Here's the drawing with two shaded views (mm, measured from the low corner). I have some questions. Round coordinates to 2 decimals unless told otherwise and drop trailing zeros. Loops run counter-clockwise (first coordinate to the right, second up) from the corner with the lowest first, then second, coordinate; pieces in that order, holes last. Notation, with made-up numbers: (63.25, 86) -> (75.25, 86) arc R22 ccw to (75.25, 105) -> close; hole circle Ø3 at (6, 56.5). An arc over 180 degrees is marked (long way). Write item = value, one per line.
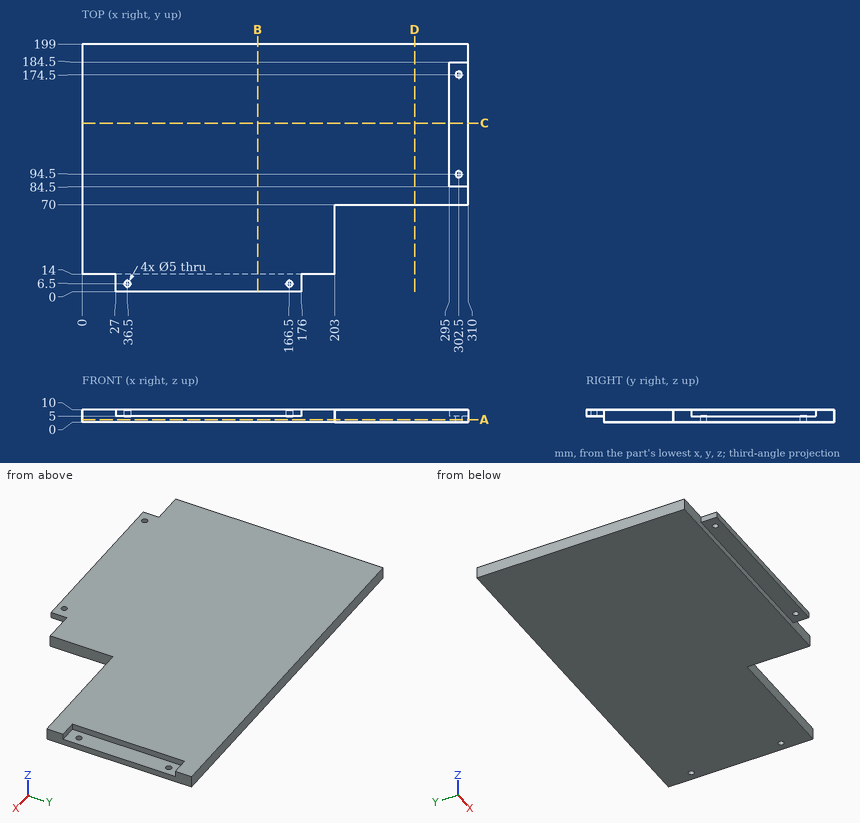
1. Suppose I cut it at A-A, the plane z = 2.25. List the corners of the cut face in (x, y) for me.
Entries:
outline = (0, 14) -> (203, 14) -> (203, 70) -> (310, 70) -> (310, 199) -> (0, 199) -> close; hole circle Ø5 at (302.5, 94.5); hole circle Ø5 at (302.5, 174.5)
2. I need wall thicknesses on line 1 (Y direction, x = 302.5, z = 1.9); line 2 (Y direction, x = 36.5, z = 8.7); line 3 (X direction, y = 144, z = 9.25). Which ranges of each line are inside material? Lowest first, please. Write a range as [from, to].
Entries:
line_1 = [70, 92], [97, 172], [177, 199]
line_2 = [0, 4], [9, 199]
line_3 = [0, 295]
3. Suppose I cut it at C-C, the plane y = 135.5. List the corners of the cut face in (x, z) for me, and give its area (4 significant figures).
Entries:
outline = (0, 0) -> (310, 0) -> (310, 5) -> (295, 5) -> (295, 10) -> (0, 10) -> close
area = 3,025 mm²
4. I'm going to push flat-ended pins straight in: pin 1 (12 mm diameter, centred on x = 303, y = 122.5, fed in from +Z); pin 2 (6 mm diameter, centred on x = 36.5, y = 6.5, fed in from -Z); pin 3 (2.5 mm diameter, centred on x = 300, z = 7.5, fed in from -Y); pin 4 (3 mm diameter, centred on x = 166.5, y = 6.5, fed in from +Z). Where does each tip first touch, or does it pass through?
Entries:
pin_1 = 5
pin_2 = 5
pin_3 = 70
pin_4 = through
5. Suppose I cut it at D-D, the plane x = 267. List the corners of the cut face in (y, z) for me.
Entries:
outline = (70, 0) -> (199, 0) -> (199, 10) -> (70, 10) -> close
6. Suppose I cut it at B-B, the plane x = 141. List the corners of the cut face in (y, z) for me, and give its area (3 significant figures).
Entries:
outline = (0, 5) -> (14, 5) -> (14, 0) -> (199, 0) -> (199, 10) -> (0, 10) -> close
area = 1,920 mm²
